Check sheet for the drawn part. Datum: minimum x, y, z corner. Units: mm. Give positions to 0.01 mm unless a question says otherwise; leave off trailing zeros. Order: outer loops, then holes, each group sorted by start corner. A loop starts at its lowest first (then second) coordinate and runs counter-clockwise, first axis right, second up. Notation, with made-up numbers: (70, 13.25) -> (104, 13.25) arc R26 cw to (104, 30.25) -> close; hole circle Ø11 at (62, -1). An arc over 180 degrees is marked (long way). Answer in a Markdown table with one row per item. Add a question column.
(1) Cross-section at A-A (y = 186). Record the cut outline in (x, z).
(2) Thickness scan on L1, parallel to X at y = 225, z = 2.1; L2, parallel to Y at x = 50.5, z = 3.7. Record the ranges inside material, lowest first. Write a range as [from, to].
(3) Go/stop test with flat-tipped pins: pin 1 (1.2 mm diameter, centred on y = 302, z = 1.5, fed in from +X); pin 2 (2 mm diameter, centred on x = 1, z = 1.5, fed in from +Y). Record where each tip stops, or that it passes through.
(4) Cross-section at B-B (z = 2.85). Record the cut outline in (x, y).
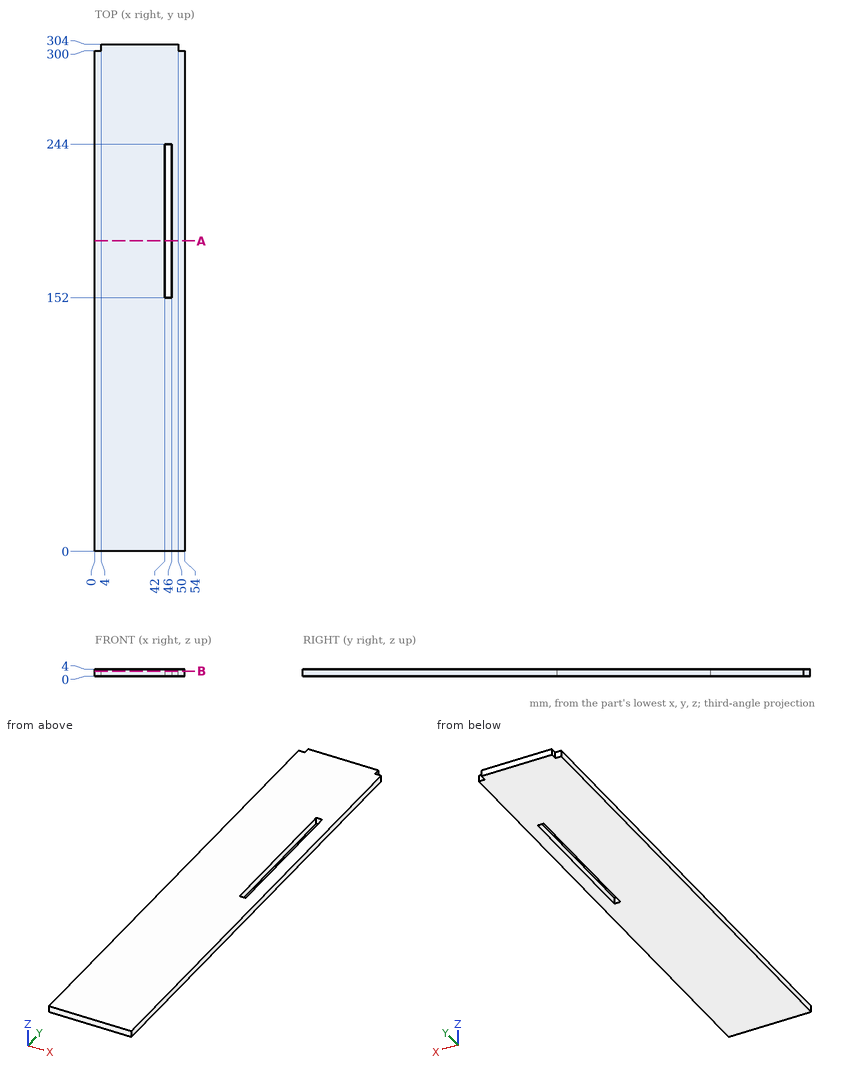
Answer below:
| question | item | result |
|---|---|---|
| 1 | outline | (0, 0) -> (42, 0) -> (42, 4) -> (0, 4) -> close; (46, 0) -> (54, 0) -> (54, 4) -> (46, 4) -> close |
| 2 | L1 | x = [0, 42], [46, 54] |
| 2 | L2 | y = [0, 300] |
| 3 | pin 1 | stops at x = 50 |
| 3 | pin 2 | stops at y = 300 |
| 4 | outline | (0, 0) -> (54, 0) -> (54, 300) -> (50, 300) -> (50, 304) -> (4, 304) -> (4, 300) -> (0, 300) -> close; hole (42, 152) -> (46, 152) -> (46, 244) -> (42, 244) -> close |
